```python
from build123d import *

# Parameters (mm, degrees)
SKETCH2_W            = 101.6
SKETCH2_H            = 6.35
BOSS_EXTRUDE1_DEPTH  = 50.8
M3_CLEARANCE_HOLE1_D = 3.4


with BuildPart() as part:
    # Sketch2 → Boss-Extrude1 (new body)
    with BuildSketch(Plane(origin=(0, 0, 0), x_dir=(1, 0, 0), z_dir=(0, 1, 0))):
        with Locations((50.8, 3.175)):
            Rectangle(SKETCH2_W, SKETCH2_H)
    extrude(amount=BOSS_EXTRUDE1_DEPTH)

    # M3 Clearance Hole1 (through all)
    with Locations(Plane.XY):
        with Locations((50.8, 17.78)):
            Hole(M3_CLEARANCE_HOLE1_D / 2)


solid = part.part
```
Verification items for the finished model (mm, model axes). Round coordinates to 2 decimals unless told otherwise and drop trailing zeros. Loops run counter-clockwise (first coordinate to the right, second up) from the corner with the lowest first, then second, coordinate; pieces in that order, holes last. Notation, with made-up numbers: (29, 21.25) -> (71, 21.25) arc R13 ccw to (71, 36.25) -> close; hole circle Ø2 at (-17.75, -36). An arc over 180 degrees is marked (long way). Answer as a JSON object with one key per item and string values.
Q1. Scan line: line 1 (Y direction, x = 50.8, z = -3.75). Record every from-to range of solid material in increasing order. Write a range as from..to.
Data:
{"line 1": "y = 0..16.08, 19.48..50.8"}
Q2. Go/stop test with flat-tipped pins: P1, Ø1, axis at x = 21.5, z = -5, coming from the -Y side; P2, Ø2, axis at x = 50.8, y = 17.78, coming from the +Z side. Record where each tip stops, or that it passes through.
Data:
{"P1": "stops at y = 0", "P2": "passes through"}
Q3. Draft check along X on faces 1 (the flat face through (50, 25, -6.35)), 2 (the flat face through (101.6, 25, -3)), 3 (the cylindrical face through (52.5, 17.85, -3.22)). Enter one of: pulls with the +X half, pulls with the -X half, needs draft (parallel to the pull), parting line crosses it, or undercut.
Data:
{"face 1": "needs draft", "face 2": "pulls with the +X half", "face 3": "undercut"}
Q4. Section check B-B (y = 17.78). Record the boundary of the cut face in (x, z), then the cut area to 3 significant figures.
Data:
{"outline": "(0, -6.35) -> (49.1, -6.35) -> (49.1, 0) -> (0, 0) -> close; (52.5, -6.35) -> (101.6, -6.35) -> (101.6, 0) -> (52.5, 0) -> close", "area": "624 mm2"}
Q5. Section check A-A (x = 50.8). Record the boundary of the cut face in (y, z), then the cut area to 3 significant figures.
Data:
{"outline": "(0, -6.35) -> (16.08, -6.35) -> (16.08, 0) -> (0, 0) -> close; (19.48, -6.35) -> (50.8, -6.35) -> (50.8, 0) -> (19.48, 0) -> close", "area": "301 mm2"}
